Autodesk Inventor part; units mm, degrees
ref_plane "YZ Plane" through (0, 0, 0) normal (1, 0, 0) x (0, 1, 0)
ref_plane "XZ Plane" through (0, 0, 0) normal (0, 1, 0) x (-1, 0, 0)
ref_plane "XY Plane" through (0, 0, 0) normal (0, 0, 1) x (1, 0, 0)
sketch "Sketch1" plane through (0, 0, 0) normal (0, 0, 1) x (1, 0, 0)
  line L0 (-50, -15) -> (50, -15)
  line L1 (50, -15) -> (50, 15)
  line L2 (50, 15) -> (-50, 15)
  line L3 (-50, 15) -> (-50, -15)
  line L4 (-50, -15) -> (50, 15) construction
  line L5 (50, -15) -> (-50, 15) construction
  point P0 (0, 0)
  dimension "d0" = 100
  dimension "d1" = 30
extrude "Extrusion1" add sketch "Sketch1" along normal blind 10
sketch "Sketch2" plane through (0, 0, 10) normal (0, 0, 1) x (1, 0, 0)
  line L0 (-50, -15) -> (50, -15)
  line L1 (50, -15) -> (50, 15)
  line L2 (50, 15) -> (-50, 15)
  line L3 (-50, 15) -> (-50, -15)
  line L4 (-45, 10) -> (45, 10)
  line L5 (45, 10) -> (45, -10)
  line L6 (45, -10) -> (-45, -10)
  line L7 (-45, -10) -> (-45, 10)
  point P0 (0, 0)
  dimension "d4" = 5
extrude "Extrusion2" cut sketch "Sketch2" against normal blind 6 contours L4 L5 L6 L7
sketch "Sketch3" plane through (0, 0, 10) normal (0, 0, 1) x (1, 0, 0)
  line L0 (-45, -10) -> (-45, 10)
  line L1 (-45, 10) -> (45, 10)
  line L2 (45, 10) -> (45, -10)
  line L3 (45, -10) -> (-45, -10)
  line L4 (-50, -15) -> (50, -15)
  line L5 (50, -15) -> (50, 15)
  line L6 (50, 15) -> (-50, 15)
  line L7 (-50, 15) -> (-50, -15)
  line L8 (-50, 15) -> (-50, -15)
  line L9 (-50, -5.5) -> (-45, -5.5)
  line L10 (-45, -5.5) -> (-45, 5.5)
  line L11 (-45, 5.5) -> (-50, 5.5)
  line L12 (-50, 5.5) -> (-50, -5.5)
  line L13 (-70, 0) -> (70, 0)
  line L14 (45, 10) -> (45, -10)
  line L15 (50, -15) -> (50, 15)
  line L16 (50, 15) -> (-50, 15)
  line L17 (-45, 10) -> (45, 10)
  line L18 (-40.5, 15) -> (-29.5, 15)
  line L19 (-29.5, 15) -> (-29.5, 10)
  line L20 (-29.5, 10) -> (-40.5, 10)
  line L21 (-40.5, 10) -> (-40.5, 15)
  line L22 (-35, 15) -> (-35, 10) construction
  line L23 (-45, 10) -> (45, 10)
  line L24 (45, -10) -> (-45, -10)
  line L25 (-50, -15) -> (50, -15)
  line L26 (-40.5, -10) -> (-29.5, -10)
  line L27 (-29.5, -10) -> (-29.5, -15)
  line L28 (-29.5, -15) -> (-40.5, -15)
  line L29 (-40.5, -15) -> (-40.5, -10)
  line L30 (45, 10) -> (45, -10)
  line L31 (45, 5.5) -> (50, 5.5)
  line L32 (50, 5.5) -> (50, -5.5)
  line L33 (50, -5.5) -> (45, -5.5)
  line L34 (45, -5.5) -> (45, 5.5)
  point P0 (0, 0)
  dimension "d7" = 11
  dimension "d9" = 11
  dimension "d10" = 15
  dimension "d28" = 11
  dimension "d29" = 11
extrude "Extrusion3" cut sketch "Sketch3" against normal blind 2 contours L9 L7 L13 L0 | L3 L27 L4 L29 | L13 L7 L11 L0 | L13 L5 L33 L2 | L2 L31 L5 L13 | L21 L6 L19 L1
sketch "Sketch4" plane through (0, 0, 10) normal (0, 0, 1) x (1, 0, 0)
  line L0 (-50, -15) -> (50, -15)
  line L1 (-50, 15) -> (-50, -15)
  line L2 (50, 15) -> (-50, 15)
  line L3 (50, -15) -> (50, 15)
  point P0 (0, 0)
  point P1 (-47.5, 12.5)
  dimension "d16" = 2.5
  dimension "d17" = 2.5
hole "Hole1" at (-47.5, 12.5, 10) direction (0, 0, -1) diameter 2.013 end through all
mirror "Mirror1" about plane through (0, 0, 0) normal (0, 1, 0) of "Hole1"
mirror "Mirror2" about plane through (0, 0, 0) normal (1, 0, 0) of "Hole1", "Mirror1"
equation "\"d9\" = d7"
equation "\"d28\" = d7"
equation "\"d29\" = d7"
properties part number "PassiveSwitchCase"
Can you work these out from the model? Positions are in its coordinate system, mm. A direction names the side the tool comes from. Coordinates: 2 decimals unless noted, no trailing zeros. Write each loop counter-clockwise with the first axis right and the second up, starting at its lowest first coordinate (ties: lowest second). Pieces come first, ordered by that corner, then holes. Notation, with made-up numbers: (56.25, 31) - (84.25, 31) arc R30 cw to (84.25, 60) - close; hole circle Ø8 at (-1.5, 41). An arc over 180 degrees is marked (long way). Return JSON: item names as keys, results as strings.
Q1. I'm going to push a flat-ended pin straight in: pin 1 Ø5.5 at (x, y) = (-47.5, -2.5) entering from +Z. Where does the tip first touch, or does it pass through?
Computed values:
{"pin 1": "stops at z = 8"}
Q2. If we section it at D-D (x = -36.5): Please give me the cut outline in (y, z), then the cut area to 3 significant figures.
Computed values:
{"outline": "(-15, 0) - (15, 0) - (15, 8) - (10, 8) - (10, 4) - (-10, 4) - (-10, 8) - (-15, 8) - close", "area": "160 mm2"}
Q3. Thinking about a two-plate mould opening in Y: for faces 1 (the flat face through (-1, -15, 5)), 2 (the flat face through (1, -10, 7)), 3 (the flat face through (10, -12, 10)), 4 (the flat face through (-48, 0, 8)), which applies, +Y half, -Y half, draft (parallel to the pull), parting line (faces both ways), or undercut?
Computed values:
{"face 1": "-Y half", "face 2": "undercut", "face 3": "draft", "face 4": "undercut"}
Q4. On a 3-axis mill with a long thin cutter (end or side, diameter ignored), from which of +Z, -Z, +X, -X, +Y, -Y can I reach the whole of each face in a straight line? I mean faces 5 (the flat face through (-48, -5.5, 9)), 6 (the flat face through (-29.5, -12, 9)), 7 (the flat face through (10, 12, 10)), 8 (the flat face through (-1, 0, 4)). Say none if no direction works.
Computed values:
{"face 5": "+Z, +X, -X", "face 6": "+Z, +Y, -Y", "face 7": "+Z, +X, -X, +Y, -Y", "face 8": "+Z"}
Q5. If we section it at A-A (y = 12.5): Please give me the cut outline in (x, z).
Computed values:
{"outline": "(-50, 0) - (-48.51, 0) - (-48.51, 10) - (-50, 10) - close; (-46.49, 0) - (46.49, 0) - (46.49, 10) - (-29.5, 10) - (-29.5, 8) - (-40.5, 8) - (-40.5, 10) - (-46.49, 10) - close; (48.51, 0) - (50, 0) - (50, 10) - (48.51, 10) - close"}
Q6. If we section it at C-C (z = 5.25): Please give me the cut outline in (x, y), then the cut area to 3 significant figures.
Computed values:
{"outline": "(-50, -15) - (50, -15) - (50, 15) - (-50, 15) - close; hole circle Ø2.01 at (-47.5, -12.5); hole circle Ø2.01 at (-47.5, 12.5); hole (-45, -10) - (45, -10) - (45, 10) - (-45, 10) - close; hole circle Ø2.01 at (47.5, -12.5); hole circle Ø2.01 at (47.5, 12.5)", "area": "1,190 mm2"}
Q7. If we section it at B-B (x = -47.5): Please give me the cut outline in (y, z), then the cut area to 3 significant figures.
Computed values:
{"outline": "(-15, 0) - (-13.51, 0) - (-13.51, 10) - (-15, 10) - close; (-11.49, 0) - (11.49, 0) - (11.49, 10) - (5.5, 10) - (5.5, 8) - (-5.5, 8) - (-5.5, 10) - (-11.49, 10) - close; (13.51, 0) - (15, 0) - (15, 10) - (13.51, 10) - close", "area": "238 mm2"}
Q8. Please list where these lines run through material, in increasing order: L1, parallel to Y at x = -47.5, z = 2.5; L2, parallel to X at y = -12.5, z = 3; L3, parallel to Y at x = -12.5, z = 8. Write a range as from..to.
Computed values:
{"L1": "y = -15..-13.51, -11.49..11.49, 13.51..15", "L2": "x = -50..-48.51, -46.49..46.49, 48.51..50", "L3": "y = -15..-10, 10..15"}
